The listing builds one solid part. Answer for the finished solid, in the listing's coordinates (mm). Coordinates: 2 decimals unless noted, no trailing zeros. Loops run counter-clockwise (first coordinate to the right, second up) from the corner with the lowest first, then second, coordinate; pieces in that order, holes last. Notation, with made-up numbers: (-28.75, 42) -> (1.25, 42) arc R20 ccw to (1.25, 53) -> close; hole circle Ø4 at (85, 78). An arc over 180 degrees is marked (long way). Answer in a Markdown table with one row per item.
```python
from build123d import *

# Parameters (mm, degrees)
SKETCH2_R          = 6.35
CUT_EXTRUDE1_DEPTH = 25.4
FILLET1_R          = 0.508


with BuildPart() as part:
    # Sketch1 → Revolve1 (revolve)
    with BuildSketch(Plane.XY):
        with BuildLine():
            Line((0, 11.1125), (0, -11.1125))
            ThreePointArc((0, -11.1125), (-11.1125, 0), (0, 11.1125))
        make_face()
    revolve(axis=Axis((0, 11.1125, 0), (0, -1, 0)))

    # Sketch2 → Cut-Extrude1 (cut, symmetric)
    with BuildSketch(Plane(origin=(0, 0, 0), x_dir=(1, 0, 0), z_dir=(0, 1, 0))):
        Circle(SKETCH2_R)
    extrude(amount=CUT_EXTRUDE1_DEPTH, both=True, mode=Mode.SUBTRACT)

    # Fillet1
    fillet1_edges = [part.edges().sort_by_distance(p)[0] for p in [
        (0, 9.119493201, -6.35),
        (0, -9.119493201, 6.35),
    ]]
    fillet(fillet1_edges, radius=FILLET1_R)


solid = part.part
```
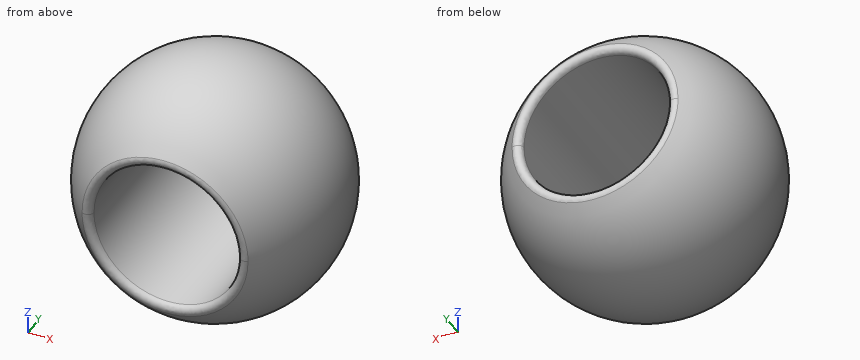
Item 1: A cutting plane is placed at D-D, the plane y = -0.25. Determine the outline of the cut face in (x, z), plus the area to 3 significant figures.
Findings below:
| item | result |
|---|---|
| outline | circle Ø22.22 at (0, 0); hole circle Ø12.7 at (0, 0) |
| area | 261 mm2 |
Item 2: A cutting plane is placed at A-A, the plane y = 2. Determine the outline of the cut face in (x, z), plus the area to 3 significant figures.
Findings below:
| item | result |
|---|---|
| outline | circle Ø21.86 at (0, 0); hole circle Ø12.7 at (0, 0) |
| area | 249 mm2 |
Item 3: Find the intervals of material crossed by probe 1 along Z at (x, y) = (0.5, 1); probe 2 along X at (y, z) = (7, -2.75); probe 3 along Z at (x, y) = (0, 2.5), in increasing order.
Findings below:
| item | result |
|---|---|
| probe 1 | z = -11.06 to -6.33, 6.33 to 11.06 |
| probe 2 | x = -8.18 to -5.72, 5.72 to 8.18 |
| probe 3 | z = -10.83 to -6.35, 6.35 to 10.83 |
Item 4: Flat-ended cylindrical pins translate along their axes: pin 1 Ø6 at (x, y) = (5.5, -5.5) entering from +Z; pin 2 Ø5 at (x, y) = (-7, -3) entering from -Z; pin 3 Ø4 at (y, z) = (-6.5, 1.5) entering from +X. Find the tip coordinate at first contact, or state that the pin passes through.
Findings below:
| item | result |
|---|---|
| pin 1 | stops at z = 10.03 |
| pin 2 | stops at z = -9.86 |
| pin 3 | stops at x = 10.08 |
Item 5: A cutting plane is placed at C-C, the plane z = 9.5. Determine the outline of the cut face in (x, y), plus the area to 3 significant figures.
Findings below:
| item | result |
|---|---|
| outline | circle Ø11.53 at (0, 0) |
| area | 104 mm2 |
Item 6: A cutting plane is placed at B-B, the plane x = 8. Determine the outline of the cut face in (y, z), plus the area to 3 significant figures.
Findings below:
| item | result |
|---|---|
| outline | circle Ø15.43 at (0, 0) |
| area | 187 mm2 |
